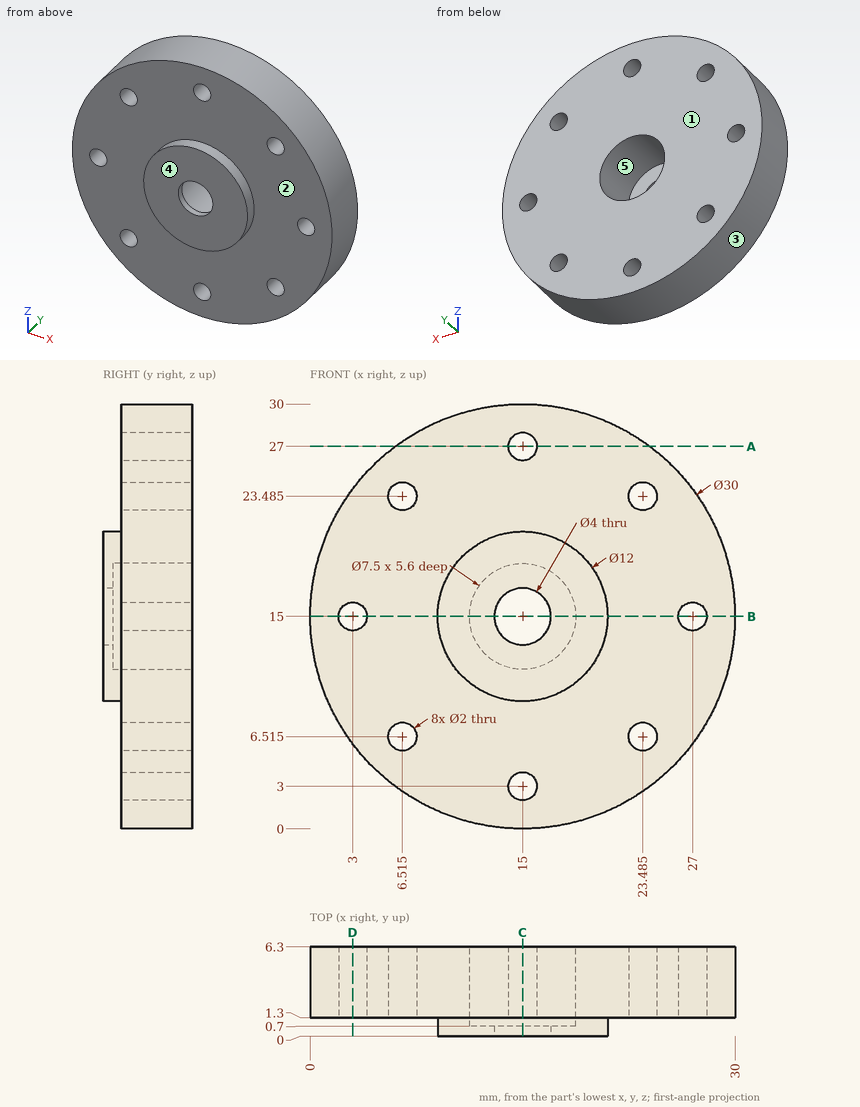
Source: three-view drawing plus pictorial views. Frame: mm from the lowest corner of the part. A direction names the side the tool comes from. Coordinates: 2 decimals unless noted, no trailing zeros. Loops run counter-clockwise (first coordinate to the right, second up) from the corner with the lowest first, then second, coordinate; pieces in that order, holes last. Notation, with made-up numbers: (16.25, -2.75) - (55.25, -2.75) arc R21 ccw to (55.25, 21.25) - close; hole circle Ø11 at (-1, 55.5). An arc over 180 degrees is marked (long way). One line per question, with ' | ' between items.
1) Section A-A, the plane z = 27. Return loops of the section in (x, y), then the cut area to 3 significant figures.
Report:
outline: (6, 1.3) - (14, 1.3) - (14, 6.3) - (6, 6.3) - close; (16, 1.3) - (24, 1.3) - (24, 6.3) - (16, 6.3) - close | area: 80.0 mm²
2) Line query: line 1 along X through (y, z) = (3.7, 15); line 2 along X through (y, z) = (4.5, 23.5) (1 decimal); line 3 along X through (y, z) = (3.5, 15.75) (1 decimal). Output: solid intervals per line, ascending.
Report:
line 1: x = 0 to 2, 4 to 11.25, 18.75 to 26, 28 to 30 | line 2: x = 2.6 to 5.5, 7.5 to 22.5, 24.5 to 27.4 | line 3: x = 0 to 2.3, 3.7 to 11.3, 18.7 to 26.3, 27.7 to 30
3) Section C-C, the plane x = 15. Return loops of the section in (y, z), then the cut area to 3 significant figures.
Report:
outline: (0, 9) - (1.3, 9) - (1.3, 4) - (6.3, 4) - (6.3, 11.25) - (0.7, 11.25) - (0.7, 13) - (0, 13) - close; (0, 17) - (0.7, 17) - (0.7, 18.75) - (6.3, 18.75) - (6.3, 26) - (1.3, 26) - (1.3, 21) - (0, 21) - close; (1.3, 0) - (6.3, 0) - (6.3, 2) - (1.3, 2) - close; (1.3, 28) - (6.3, 28) - (6.3, 30) - (1.3, 30) - close | area: 101 mm²
4) Set-up query: the marked faces 1 and 2. Return all of +Z, -Z, +X, -X, +Y, -Y with unobstructed straight access to the full face (end or side cutting, diameter ignored); none if empty.
Report:
face 1: +Z, -Z, +X, -X, +Y | face 2: -Y
5) Section D-D, the plane x = 3. Return loops of the section in (y, z), then the cut area to 3 significant figures.
Report:
outline: (1.3, 6) - (6.3, 6) - (6.3, 14) - (1.3, 14) - close; (1.3, 16) - (6.3, 16) - (6.3, 24) - (1.3, 24) - close | area: 80.0 mm²
6) Section B-B, the plane z = 15. Return loops of the section in (x, y).
Report:
outline: (0, 1.3) - (2, 1.3) - (2, 6.3) - (0, 6.3) - close; (4, 1.3) - (9, 1.3) - (9, 0) - (13, 0) - (13, 0.7) - (11.25, 0.7) - (11.25, 6.3) - (4, 6.3) - close; (17, 0) - (21, 0) - (21, 1.3) - (26, 1.3) - (26, 6.3) - (18.75, 6.3) - (18.75, 0.7) - (17, 0.7) - close; (28, 1.3) - (30, 1.3) - (30, 6.3) - (28, 6.3) - close
7) Pull-direction query (Z, two-part tool) for the marked faces 3, 4 and 5; classes: released by +Z, released by -Z, zero draft, split by the parting line, or undercut.
Report:
face 3: split by the parting line | face 4: zero draft | face 5: undercut
8) First-contact query: P1, Ø1.2, axis at x = 6.51, z = 6.51, coming from the -Y side; P2, Ø1.5, axis at x = 4, y = 1.5, coming from the -Z side; P3, Ø3, axis at x = 23.49, z = 23.49, coming from the -Y side; P4, Ø2, axis at y = 2, z = 17.5, coming from the +X side (1 decimal). Flat tips, straight axial feed; report the tip coordinate or a pass-through.
Report:
P1: passes through | P2: stops at z = 4.05 | P3: stops at y = 1.3 | P4: stops at x = 29.9
